from build123d import *

# Parameters (mm, degrees)
SKETCH2_R           = 1.984375
SKETCH2_W           = 39.6875
SKETCH2_H           = 19.05
BOSS_EXTRUDE1_DEPTH = 6.35


with BuildPart() as part:
    # Sketch2 → Boss-Extrude1 (new body)
    with BuildSketch(Plane.XY):
        Polygon((51.59375, 25.4), (-11.90625, 25.4), (-11.90625, -19.05), (0.79375, -19.05), (0.79375, -12.7), (13.49375, -12.7), (13.49375, -19.05), (26.19375, -19.05), (26.19375, -12.7), (38.89375, -12.7), (38.89375, -19.05), (51.59375, -19.05), align=None)
        with Locations((-3.96875, 4.525)):
            Circle(SKETCH2_R, mode=Mode.SUBTRACT)
        with Locations((-3.96875, 14.525)):
            Circle(SKETCH2_R, mode=Mode.SUBTRACT)
        with Locations((19.84375, 9.525)):
            Rectangle(SKETCH2_W, SKETCH2_H, mode=Mode.SUBTRACT)
        with Locations((43.65625, 4.525)):
            Circle(SKETCH2_R, mode=Mode.SUBTRACT)
        with Locations((43.65625, 14.525)):
            Circle(SKETCH2_R, mode=Mode.SUBTRACT)
    extrude(amount=BOSS_EXTRUDE1_DEPTH)


solid = part.part
Source: CAD feature listing. Evaluate the final solid. Frame: model axes, mm. A direction names the side the tool comes from. Give positions to 0.01 mm unless a question says otherwise; leave off trailing zeros. Order: outer loops, then holes, each group sorted by start corner. A loop starts at its lowest first (then second) coordinate and runs counter-clockwise, first axis right, second up. Notation, with made-up numbers: (-21, 5) -> (-11, 5) arc R13 cw to (-11, 13) -> close; hole circle Ø3 at (11, -22). An arc over 180 degrees is marked (long way). Use a Markdown table: item, result.
1) Section query D-D, the plane z = 5.25. Count the separate pieces of the cut face and the enclosed holes in it, then the cut area to 3 significant figures.
Answer list:
| item | result |
|---|---|
| separate pieces | 1 |
| enclosed holes | 5 |
| area | 1,860 mm² |
2) Section query C-C, the plane y = -15.5. Return the cut outline in (x, z).
Answer list:
| item | result |
|---|---|
| outline | (-11.91, 0) -> (0.79, 0) -> (0.79, 6.35) -> (-11.91, 6.35) -> close; (13.49, 0) -> (26.19, 0) -> (26.19, 6.35) -> (13.49, 6.35) -> close; (38.89, 0) -> (51.59, 0) -> (51.59, 6.35) -> (38.89, 6.35) -> close |
3) Ray query, line 1 along X through (y, z) = (-16, 2.5); line 2 along Y through (x, z) = (2.5, 2); line 3 along X through (y, z) = (4.5, 0.75). Return the intervals inside material, ascending. Write a range as [from, to].
Answer list:
| item | result |
|---|---|
| line 1 | [-11.91, 0.79], [13.49, 26.19], [38.89, 51.59] |
| line 2 | [-12.7, 0], [19.05, 25.4] |
| line 3 | [-11.91, -5.95], [-1.98, 0], [39.69, 41.67], [45.64, 51.59] |
4) Section query A-A, the plane x = 11. Return the cut outline in (y, z), then the cut area to 3 significant figures.
Answer list:
| item | result |
|---|---|
| outline | (-12.7, 0) -> (0, 0) -> (0, 6.35) -> (-12.7, 6.35) -> close; (19.05, 0) -> (25.4, 0) -> (25.4, 6.35) -> (19.05, 6.35) -> close |
| area | 121 mm² |
5) Section query B-B, the plane y = 11.5. Return the cut outline in (x, z).
Answer list:
| item | result |
|---|---|
| outline | (-11.91, 0) -> (0, 0) -> (0, 6.35) -> (-11.91, 6.35) -> close; (39.69, 0) -> (51.59, 0) -> (51.59, 6.35) -> (39.69, 6.35) -> close |
6) Reachability of faces 1 (the flat face through (13.494, -16, 3)), 2 (the flat face through (-11.906, 3, 3)), 3 (the flat face through (0, 9, 3)) from +Z, -Z, +X, -X, +Y, -Y: full face, straight path, thin tool, end or side. Return the list, or none.
Answer list:
| item | result |
|---|---|
| face 1 | +Z, -Z, -Y |
| face 2 | +Z, -Z, -X, +Y, -Y |
| face 3 | +Z, -Z |
7) Contact query for flat-ended pins moving along their axis: P1, Ø5, axis at x = 43.66, y = 14.52, coming from the +Z side; P2, Ø3, axis at x = 9, z = 2, coming from the -Y side. Output: stop coordinate, or through.
Answer list:
| item | result |
|---|---|
| P1 | z = 6.35 |
| P2 | y = -12.7 |
8) Mould query, pull axis Y, two halves, no side actions, for faces 4 (the cylindrical face through (-5.95, 4.61, 3.13)), 5 (the flat face through (-6, -19.05, 3)), 6 (the flat face through (19, -1, 0)), 7 (the flat face through (20, 25.4, 3)). Classes: +Y half, -Y half, draft (parallel to the pull), parting line (faces both ways), or undercut.
Answer list:
| item | result |
|---|---|
| face 4 | undercut |
| face 5 | -Y half |
| face 6 | draft |
| face 7 | +Y half |
